```python
from build123d import *

# Parameters (mm, degrees)
SKETCH1_R           = 10.2
BOSS_EXTRUDE1_DEPTH = 25.1
SKETCH2_R           = 10
BOSS_EXTRUDE2_DEPTH = 18.5
SKETCH3_R           = 3.5
BOSS_EXTRUDE3_DEPTH = 3
SKETCH4_R           = 2
BOSS_EXTRUDE4_DEPTH = 10.5
CUT_EXTRUDE1_DEPTH  = 10.5
SKETCH6_R           = 1.25
CUT_EXTRUDE2_DEPTH  = 3


with BuildPart() as part:
    # Sketch1 → Boss-Extrude1 (new body)
    with BuildSketch(Plane(origin=(0, 0, 0), x_dir=(0, 0, -1), z_dir=(1, 0, 0))):
        Circle(SKETCH1_R)
    extrude(amount=BOSS_EXTRUDE1_DEPTH)

    # Sketch2 → Boss-Extrude2 (add)
    with BuildSketch(Plane.ZY):
        with Locations(Location((0, 0, 0), (0, 0, 180))):
            Circle(SKETCH2_R)
    extrude(amount=BOSS_EXTRUDE2_DEPTH)

    # Sketch3 → Boss-Extrude3 (add)
    with BuildSketch(Plane.ZY.offset(18.5)):
        Circle(SKETCH3_R)
    extrude(amount=BOSS_EXTRUDE3_DEPTH)

    # Sketch4 → Boss-Extrude4 (add)
    with BuildSketch(Plane.ZY.offset(21.5)):
        with Locations(Location((0, 0, 0), (0, 0, 180))):
            Circle(SKETCH4_R)
    extrude(amount=BOSS_EXTRUDE4_DEPTH)

    # Sketch5 → Cut-Extrude1 (cut)
    with BuildSketch(Plane.ZY.offset(32)):
        Polygon((-44.16593662, 1.5), (-1.322875656, 1.5), (1.322875656, 1.5), (44.16593662, 1.5), (44.16593662, 87.186121928), (-44.16593662, 87.186121928), align=None)
    extrude(amount=-CUT_EXTRUDE1_DEPTH, mode=Mode.SUBTRACT)

    # Sketch6 → Cut-Extrude2 (cut)
    with BuildSketch(Plane.ZY.offset(18.5)):
        with Locations((0, 7.5)):
            Circle(SKETCH6_R)
        with Locations((0, -7.5)):
            Circle(SKETCH6_R)
    extrude(amount=-CUT_EXTRUDE2_DEPTH, mode=Mode.SUBTRACT)


solid = part.part
```
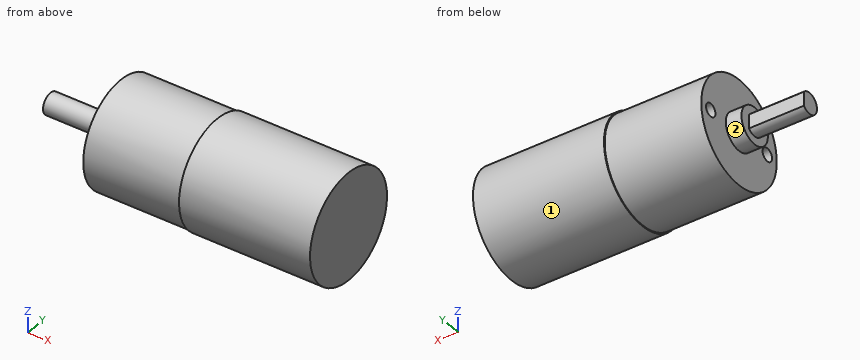
Geometry check sheet. Reference: the model listing, model coordinates, mm. Face numbers are marked on the shaded views. A direction names the side the tool comes from. Give positions to 0.01 mm unless a question says otherwise; leave off trailing zeros. Write each loop counter-clockwise with the first axis right and the second up, starting at its lowest first coordinate (ties: lowest second). Pieces come first, ordered by that corner, then holes.
1) Access from +Z, -Z, +X, -X, +Y, -Y to the whole of each face (thin tool, end or side, straight path). Record for the marked faces 1 and 2.
2) Material ranges on L1, parallel to Y at x = -17.65, z = 0; L2, parallel to Z at x = 1, y = -5.25; L3, parallel to X at y = 2.25, z = 3, recorded low to high.
3) Gauge pin test, flat ends, axial feed: pin 1 (4 mm diameter, centred on y = 7.5, z = -7, fed in from +X); pin 2 (3 mm diameter, centred on y = -7, z = 0, fed in from -X); pin 3 (1.5 mm diameter, centred on x = 14.5, z = -2.5, fed in from +Y); pin 4 (4 mm diameter, centred on x = 4.5, y = 2.5, fed in from +Z). Record the tip position at first contact, or that the pin passes through.
4) Section check B-B, the plane z = 0. Record the boundary of the cut face in (x, y), and give its area (3 significant figures).
5) Section check A-A, the plane y = 0. Record the boundary of the cut face in (x, z), and give its area (3 significant figures).
6) Section check D-D, the plane y = -7.5. Record the boundary of the cut face in (x, z), and give its area (3 significant figures).
7) Section check C-C, the plane x = 20. Record the boundary of the cut face in (y, z), and give its area (3 significant figures).
Computed:
1. face 1: +X, -X
1. face 2: -X
2. L1: y = -10 to -8.75, -6.25 to 6.25, 8.75 to 10
2. L2: z = -8.75 to 8.75
2. L3: x = -18.5 to 25.1
3. pin 1: stops at x = 25.1
3. pin 2: stops at x = -18.5
3. pin 3: stops at y = 10.05
3. pin 4: stops at z = 10.19
4. outline: (-32, -2) - (-21.5, -2) - (-21.5, -3.5) - (-18.5, -3.5) - (-18.5, -6.25) - (-15.5, -6.25) - (-15.5, -8.75) - (-18.5, -8.75) - (-18.5, -10) - (0, -10) - (0, -10.2) - (25.1, -10.2) - (25.1, 10.2) - (0, 10.2) - (0, 10) - (-18.5, 10) - (-18.5, 8.75) - (-15.5, 8.75) - (-15.5, 6.25) - (-18.5, 6.25) - (-18.5, 3.5) - (-21.5, 3.5) - (-21.5, 1.5) - (-32, 1.5) - close
4. area: 925 mm2
5. outline: (-32, -2) - (-21.5, -2) - (-21.5, -3.5) - (-18.5, -3.5) - (-18.5, -10) - (0, -10) - (0, -10.2) - (25.1, -10.2) - (25.1, 10.2) - (0, 10.2) - (0, 10) - (-18.5, 10) - (-18.5, 3.5) - (-21.5, 3.5) - (-21.5, 2) - (-32, 2) - close
5. area: 945 mm2
6. outline: (-18.5, -6.61) - (0, -6.61) - (0, -6.91) - (25.1, -6.91) - (25.1, 6.91) - (0, 6.91) - (0, 6.61) - (-18.5, 6.61) - (-18.5, 1.25) - (-15.5, 1.25) - (-15.5, -1.25) - (-18.5, -1.25) - close
6. area: 584 mm2
7. outline: circle Ø20.4 at (0, 0)
7. area: 327 mm2
